```python
from build123d import *

# Parameters (mm, degrees)
SKETCH_1_R             = 62.5
EXTRUDE_1_DEPTH        = 50
CUT_EXTRUDE_START      = -7
SKETCH_2_R             = 62.5
SKETCH_2_R_2           = 57.5
CUT_EXTRUDE_1_DEPTH    = 6
PATTERN_LINEAR_1_COUNT = 3
PATTERN_LINEAR_1_PITCH = 15
SKETCH_3_R             = 62.5
SKETCH_3_R_2           = 57.5
CUT_EXTRUDE_2_DEPTH    = 2
SKETCH_4_R             = 62.5
SKETCH_4_R_2           = 57.5
CUT_EXTRUDE_3_DEPTH    = 2
SKETCH_5_R             = 12.5
CUT_EXTRUDE_4_DEPTH    = 51


with BuildPart() as part:
    # 草图1 → 凸台-拉伸1 (new body)
    with BuildSketch(Plane(origin=(0, 0, 0), x_dir=(1, 0, 0), z_dir=(0, 1, 0))):
        Circle(SKETCH_1_R)
    extrude(amount=EXTRUDE_1_DEPTH)

    # 草图2 → 切除-拉伸1 (cut)
    with BuildSketch(Plane(origin=(0, 50, 0), x_dir=(1, 0, 0), z_dir=(0, 1, 0)).offset(CUT_EXTRUDE_START)):
        Circle(SKETCH_2_R)
        Circle(SKETCH_2_R_2, mode=Mode.SUBTRACT)
    cut_extrude_1 = extrude(amount=-CUT_EXTRUDE_1_DEPTH, mode=Mode.SUBTRACT)

    # 阵列(线性)1: 切除-拉伸1 ×3
    with Locations(*[(0, -i * PATTERN_LINEAR_1_PITCH, 0) for i in range(1, PATTERN_LINEAR_1_COUNT)]):
        add(cut_extrude_1, mode=Mode.SUBTRACT)

    # 草图3 → 切除-拉伸2 (cut)
    with BuildSketch(Plane(origin=(0, 50, 0), x_dir=(1, 0, 0), z_dir=(0, 1, 0))):
        Circle(SKETCH_3_R)
        Circle(SKETCH_3_R_2, mode=Mode.SUBTRACT)
    extrude(amount=-CUT_EXTRUDE_2_DEPTH, mode=Mode.SUBTRACT)

    # 草图4 → 切除-拉伸3 (cut)
    with BuildSketch(Plane.XZ):
        Circle(SKETCH_4_R)
        Circle(SKETCH_4_R_2, mode=Mode.SUBTRACT)
    extrude(amount=-CUT_EXTRUDE_3_DEPTH, mode=Mode.SUBTRACT)

    # 草图5 → 切除-拉伸4 (cut, through all)
    with BuildSketch(Plane(origin=(0, 50, 0), x_dir=(1, 0, 0), z_dir=(0, 1, 0))):
        Circle(SKETCH_5_R)
    extrude(amount=-CUT_EXTRUDE_4_DEPTH, mode=Mode.SUBTRACT)


solid = part.part
```
Model file for the job. Use its own axes, mm. A direction names the side the tool comes from. Coordinates: 2 decimals unless noted, no trailing zeros. Write each loop counter-clockwise with the first axis right and the second up, starting at its lowest first coordinate (ties: lowest second). Pieces come first, ordered by that corner, then holes. Notation, with made-up numbers: (39, 72) - (69, 72) arc R16 ccw to (69, 89) - close; hole circle Ø4 at (9, 1.25). An arc over 180 degrees is marked (long way). Use a Markdown table: item, result. Add a question column.
Item 1: 3-axis set-ups, long thin cutter, end or side, ignore diameter. For faces 4 (the face through (27, 48, 51)), 5 (the face through (27, 2, -51)), 6 (the face through (27, 22, 51)): which of +Z, -Z, +X, -X, +Y, -Y reach the whole face in a straight line?
Item 2: Band-saw the part on B-B, the plane y = 26.5. Write the cut outline in (x, z).
Item 3: Band-saw the part on A-A, the plane y = 18.5. Write the cut outline in (x, z), and give its area (3 significant figures).
Item 4: Drop flat-ended pins along their axis: pin 1 (3 mm diameter, centred on y = 13.5, z = 14, fed in from -X); pin 2 (2 mm diameter, centred on y = 24.5, z = -19, fed in from +X); pin 3 (20 mm diameter, centred on x = 0, z = 0, fed in from -Y); pin 4 (1.5 mm diameter, centred on y = 14.5, z = -6.5, fed in from -X). Give the stop position or say it passes through.
Item 5: Drill centre lines: line 1 along Y through (x, z) = (-48, 33); line 2 along X through (y, z) = (38, 0). Where is each one in solid material? Low to high.
Item 6: Two-plate mould, pull along Z, no slides. Class faces 1 (the face through (11.923, 25.35, -3.755)), 2 (the face through (-12.465, 40.042, 56.133)), 3 (the face through (27, 28, 51)): pulls with the +Z half, pulls with the -Z half, needs draft (parallel to the pull), parting line crosses it, or undercut.
A:
| question | item | result |
|---|---|---|
| 1 | face 4 | +Y |
| 1 | face 5 | -Y |
| 1 | face 6 | none |
| 2 | outline | circle Ø115 at (0, 0); hole circle Ø25 at (0, 0) |
| 3 | outline | circle Ø125 at (0, 0); hole circle Ø25 at (0, 0) |
| 3 | area | 11,800 mm² |
| 4 | pin 1 | stops at x = -61.24 |
| 4 | pin 2 | stops at x = 54.61 |
| 4 | pin 3 | passes through |
| 4 | pin 4 | stops at x = -62.23 |
| 5 | line 1 | y = 2 to 7, 13 to 22, 28 to 37, 43 to 48 |
| 5 | line 2 | x = -57.5 to -12.5, 12.5 to 57.5 |
| 6 | face 1 | undercut |
| 6 | face 2 | parting line crosses it |
| 6 | face 3 | needs draft |
